```python
from build123d import *

# Parameters (mm, degrees)
SKETCH1_W           = 355.325
SKETCH1_H           = 30
SKETCH1_R           = 12.5
SKETCH1_R_2         = 1
SKETCH1_W_2         = 50
SKETCH1_H_2         = 5
BOSS_EXTRUDE3_DEPTH = 13
FILLET3_R           = 5
SKETCH3_R           = 12.5
BOSS_EXTRUDE4_DEPTH = 13
CUT_EXTRUDE1_REACH  = 359.536
SKETCH4_R           = 1.425
SKETCH5_W           = 63.83
SKETCH5_H           = 18
CUT_EXTRUDE3_DEPTH  = 358.535810269
FILLET4_R           = 5
SKETCH6_W           = 63.8325
SKETCH6_H           = 17
CUT_EXTRUDE4_DEPTH  = 5
SKETCH7_R           = 2.159563788
SKETCH7_R_2         = 1
SKETCH7_R_3         = 2.117135705
SKETCH7_R_4         = 1.916104153
SKETCH7_R_5         = 2.415941568
BOSS_EXTRUDE5_DEPTH = 8
SKETCH8_R           = 12.5
BOSS_EXTRUDE6_DEPTH = 13
SKETCH10_W          = 20
SKETCH10_H          = 10
SKETCH10_R          = 12.5
CUT_EXTRUDE6_DEPTH  = 358.535810269
SKETCH11_R          = 13.25
CUT_EXTRUDE7_DEPTH  = 289.073524686
SKETCH12_R          = 1.25
CUT_EXTRUDE8_DEPTH  = 289.567766088
SKETCH15_R          = 1.6
CUT_EXTRUDE10_DEPTH = 292.788203368
SKETCH17_R          = 4
CUT_EXTRUDE11_DEPTH = 7.5
SKETCH18_R          = 4.25
CUT_EXTRUDE12_DEPTH = 7.5
SKETCH19_W          = 52.537451678
SKETCH19_H          = 17.901984435
CUT_EXTRUDE13_DEPTH = 5
CUT_EXTRUDE14_START = -5
SKETCH20_R          = 12.5
CUT_EXTRUDE14_DEPTH = 5


with BuildPart() as part:
    # Sketch1 → Boss-Extrude3 (new body)
    # profile 1 of 3: a face of its own
    with BuildSketch(Plane.XY):
        with Locations((177.6625, 15)):
            Rectangle(SKETCH1_W, SKETCH1_H)
        with Locations(Location((334.55, 14.5, 0), (0, 0, 180))):
            Circle(SKETCH1_R, mode=Mode.SUBTRACT)
        with Locations(Location((20.775, 14.5, 0), (0, 0, 180))):
            Circle(SKETCH1_R, mode=Mode.SUBTRACT)
    # profile 2 of 3: a face of its own
    with BuildSketch(Plane.XY):
        Polygon((177.6625, 0), (50, 0), (50, -5), (50, -17), (177.6625, -17), align=None)
        with Locations(Location((60, -14.5, 0), (0, 0, 180))):
            Circle(SKETCH1_R_2, mode=Mode.SUBTRACT)
        with Locations(Location((68, -14.5, 0), (0, 0, 180))):
            Circle(SKETCH1_R_2, mode=Mode.SUBTRACT)
        with Locations(Location((60, -2.5, 0), (0, 0, 180))):
            Circle(SKETCH1_R_2, mode=Mode.SUBTRACT)
        with Locations(Location((68, -2.5, 0), (0, 0, 180))):
            Circle(SKETCH1_R_2, mode=Mode.SUBTRACT)
    # profile 3 of 3: a face of its own
    with BuildSketch(Plane.XY):
        with Locations((25, -2.5)):
            Rectangle(SKETCH1_W_2, SKETCH1_H_2)
    extrude(amount=BOSS_EXTRUDE3_DEPTH)

    # Fillet3
    fillet3_edges = [part.edges().sort_by_distance(p)[0] for p in [
        (0, -5, 6.5),
        (0, 30, 6.5),
        (355.325, 30, 6.5),
        (355.325, 0, 6.5),
        (177.6625, -17, 6.5),
        (50, -17, 6.5),
    ]]
    fillet(fillet3_edges, radius=FILLET3_R)

    # Sketch3 → Boss-Extrude4 (add)
    with BuildSketch(Plane.XY.offset(13)):
        with Locations(Location((85, 14.5, 0), (0, 0, 180))):
            Circle(SKETCH3_R)
        with Locations(Location((165, 14.5, 0), (0, 0, 180))):
            Circle(SKETCH3_R)
        with Locations(Location((245, 14.5, 0), (0, 0, 180))):
            Circle(SKETCH3_R)
    extrude(amount=BOSS_EXTRUDE4_DEPTH)

    # Sketch4 → Cut-Extrude1 (cut, up to next)
    with BuildSketch(Plane(origin=(0, 0, 0), x_dir=(-1, 0, 0), z_dir=(0, 0, -1)), mode=Mode.PRIVATE) as cut_extrude1_sk1:
        with Locations((-68, -2.5)):
            Circle(SKETCH4_R)
    cut_extrude1_tool1 = extrude(cut_extrude1_sk1.sketch, amount=-CUT_EXTRUDE1_REACH, mode=Mode.PRIVATE) & part.part
    # Sketch4 → Cut-Extrude1 (cut, up to next)
    with BuildSketch(Plane(origin=(0, 0, 0), x_dir=(-1, 0, 0), z_dir=(0, 0, -1)), mode=Mode.PRIVATE) as cut_extrude1_sk2:
        with Locations((-60, -2.5)):
            Circle(SKETCH4_R)
    cut_extrude1_tool2 = extrude(cut_extrude1_sk2.sketch, amount=-CUT_EXTRUDE1_REACH, mode=Mode.PRIVATE) & part.part
    # Sketch4 → Cut-Extrude1 (cut, up to next)
    with BuildSketch(Plane(origin=(0, 0, 0), x_dir=(-1, 0, 0), z_dir=(0, 0, -1)), mode=Mode.PRIVATE) as cut_extrude1_sk3:
        with Locations((-60, -14.5)):
            Circle(SKETCH4_R)
    cut_extrude1_tool3 = extrude(cut_extrude1_sk3.sketch, amount=-CUT_EXTRUDE1_REACH, mode=Mode.PRIVATE) & part.part
    # Sketch4 → Cut-Extrude1 (cut, up to next)
    with BuildSketch(Plane(origin=(0, 0, 0), x_dir=(-1, 0, 0), z_dir=(0, 0, -1)), mode=Mode.PRIVATE) as cut_extrude1_sk4:
        with Locations((-68, -14.5)):
            Circle(SKETCH4_R)
    cut_extrude1_tool4 = extrude(cut_extrude1_sk4.sketch, amount=-CUT_EXTRUDE1_REACH, mode=Mode.PRIVATE) & part.part
    add(cut_extrude1_tool1.solids().sort_by_distance((68, -2.5, 0))[0], mode=Mode.SUBTRACT)
    add(cut_extrude1_tool2.solids().sort_by_distance((60, -2.5, 0))[0], mode=Mode.SUBTRACT)
    add(cut_extrude1_tool3.solids().sort_by_distance((60, -14.5, 0))[0], mode=Mode.SUBTRACT)
    add(cut_extrude1_tool4.solids().sort_by_distance((68, -14.5, 0))[0], mode=Mode.SUBTRACT)

    # Sketch5 → Cut-Extrude3 (cut, through all)
    with BuildSketch(Plane(origin=(0, 0, 0), x_dir=(-1, 0, 0), z_dir=(0, 0, -1))):
        with Locations((-145.7475, -9)):
            Rectangle(SKETCH5_W, SKETCH5_H)
    extrude(amount=-CUT_EXTRUDE3_DEPTH, mode=Mode.SUBTRACT)

    # Fillet4
    fillet4_edges = [part.edges().sort_by_distance(p)[0] for p in [
        (113.8325, -17, 6.5),
    ]]
    fillet(fillet4_edges, radius=FILLET4_R)

    # Sketch6 → Cut-Extrude4 (cut)
    with BuildSketch(Plane.XY.offset(13)):
        with Locations((81.91625, -8.5)):
            Rectangle(SKETCH6_W, SKETCH6_H)
    extrude(amount=-CUT_EXTRUDE4_DEPTH, mode=Mode.SUBTRACT)

    # Sketch7 → Boss-Extrude5 (add)
    # profile 1 of 4: a face of its own
    with BuildSketch(Plane.XY.offset(8)):
        with Locations((60, -14.5)):
            Circle(SKETCH7_R)
        with Locations((60, -14.5)):
            Circle(SKETCH7_R_2, mode=Mode.SUBTRACT)
    # profile 2 of 4: a face of its own
    with BuildSketch(Plane.XY.offset(8)):
        with Locations((60, -2.5)):
            Circle(SKETCH7_R_3)
        with Locations((60, -2.5)):
            Circle(SKETCH7_R_2, mode=Mode.SUBTRACT)
    # profile 3 of 4: a face of its own
    with BuildSketch(Plane.XY.offset(8)):
        with Locations((68, -2.5)):
            Circle(SKETCH7_R_4)
        with Locations((68, -2.5)):
            Circle(SKETCH7_R_2, mode=Mode.SUBTRACT)
    # profile 4 of 4: a face of its own
    with BuildSketch(Plane.XY.offset(8)):
        with Locations((68, -14.5)):
            Circle(SKETCH7_R_5)
        with Locations((68, -14.5)):
            Circle(SKETCH7_R_2, mode=Mode.SUBTRACT)
    extrude(amount=-BOSS_EXTRUDE5_DEPTH)

    # Sketch8 → Boss-Extrude6 (add)
    with BuildSketch(Plane.XY.offset(26)):
        with Locations(Location((85, 14.5, 0), (0, 0, 180))):
            Circle(SKETCH8_R)
        with Locations(Location((165, 14.5, 0), (0, 0, 180))):
            Circle(SKETCH8_R)
        with Locations(Location((245, 14.5, 0), (0, 0, 180))):
            Circle(SKETCH8_R)
    extrude(amount=BOSS_EXTRUDE6_DEPTH)

    # Sketch10 → Cut-Extrude6 (cut, through all)
    # profile 1 of 2: a face of its own
    with BuildSketch(Plane.XY.offset(13)):
        with Locations((275.325, 15)):
            Rectangle(SKETCH10_W, SKETCH10_H)
    # profile 2 of 2: a face of its own
    with BuildSketch(Plane.XY.offset(13)):
        with BuildLine():
            ThreePointArc((355.325, 25), (353.860533906, 28.535533906), (350.325, 30))
            Line((350.325, 30), (285.325, 30))
            Line((285.325, 30), (285.325, 20))
            Line((285.325, 20), (285.325, 10))
            Line((285.325, 10), (285.325, 0))
            Line((285.325, 0), (350.325, 0))
            ThreePointArc((350.325, 0), (353.860533906, 1.464466094), (355.325, 5))
            Line((355.325, 5), (355.325, 25))
        make_face()
        with Locations((334.55, 14.5)):
            Circle(SKETCH10_R, mode=Mode.SUBTRACT)
    extrude(amount=-CUT_EXTRUDE6_DEPTH, mode=Mode.SUBTRACT)

    # Sketch11 → Cut-Extrude7 (cut, through all)
    with BuildSketch(Plane.XY.offset(13)):
        with Locations((20.775, 14.5)):
            Circle(SKETCH11_R)
    extrude(amount=-CUT_EXTRUDE7_DEPTH, mode=Mode.SUBTRACT)

    # Sketch12 → Cut-Extrude8 (cut, through all)
    with BuildSketch(Plane.XY.offset(8)):
        with Locations((60, -2.5)):
            Circle(SKETCH12_R)
        with Locations((68, -2.5)):
            Circle(SKETCH12_R)
        with Locations((68, -14.5)):
            Circle(SKETCH12_R)
        with Locations((60, -14.5)):
            Circle(SKETCH12_R)
    extrude(amount=-CUT_EXTRUDE8_DEPTH, mode=Mode.SUBTRACT)

    # Sketch15 → Cut-Extrude10 (cut, through all)
    with BuildSketch(Plane(origin=(0, 30, 0), x_dir=(1, 0, 0), z_dir=(0, 1, 0))):
        with Locations(Location((275.325, -6.5, 0), (0, 0, 180))):
            Circle(SKETCH15_R)
    extrude(amount=-CUT_EXTRUDE10_DEPTH, mode=Mode.SUBTRACT)

    # Sketch17 → Cut-Extrude11 (cut)
    with BuildSketch(Plane(origin=(0, 30, 0), x_dir=(1, 0, 0), z_dir=(0, 1, 0))):
        with Locations(Location((275.325, -6.5, 0), (0, 0, 180))):
            Circle(SKETCH17_R)
    extrude(amount=-CUT_EXTRUDE11_DEPTH, mode=Mode.SUBTRACT)

    # Sketch18 → Cut-Extrude12 (cut)
    with BuildSketch(Plane.XZ):
        with Locations(Location((275.325, 6.5, 0), (0, 0, 270))):
            Circle(SKETCH18_R)
    extrude(amount=-CUT_EXTRUDE12_DEPTH, mode=Mode.SUBTRACT)

    # Sketch19 → Cut-Extrude13 (cut)
    with BuildSketch(Plane.XY.offset(13)):
        with Locations((23.731274161, -8.950992218)):
            Rectangle(SKETCH19_W, SKETCH19_H)
    extrude(amount=-CUT_EXTRUDE13_DEPTH, mode=Mode.SUBTRACT)

    # Sketch20 → Cut-Extrude14 (cut)
    with BuildSketch(Plane.XY.offset(39).offset(CUT_EXTRUDE14_START)):
        with Locations(Location((85, 14.5, 0), (0, 0, 180))):
            Circle(SKETCH20_R)
        with Locations(Location((165, 14.5, 0), (0, 0, 180))):
            Circle(SKETCH20_R)
        with Locations(Location((245, 14.5, 0), (0, 0, 180))):
            Circle(SKETCH20_R)
    extrude(amount=CUT_EXTRUDE14_DEPTH, mode=Mode.SUBTRACT)


solid = part.part
```
Check sheet for the modelled part. Datum: model origin and axes. Units: mm. A direction names the side the tool comes from. Coordinates: 2 decimals unless noted, no trailing zeros. Order: outer loops, then holes, each group sorted by start corner. A loop starts at its lowest first (then second) coordinate and runs counter-clockwise, first axis right, second up. Notation, with made-up numbers: (-16, 87.25) -> (0, 87.25) arc R36 ccw to (0, 126.25) -> close; hole circle Ø4 at (-22.5, 67). An arc over 180 degrees is marked (long way). Write each question's results on one line, items separated by ' | '. Start each with the question number.
1) Depth check by flat-ended pin: pin 1 (6.5 mm diameter, centred on x = 275, z = 9, fed in from +Y); pin 2 (7.5 mm diameter, centred on x = 275.325, z = 6.5, fed in from +Y); pin 3 (9 mm diameter, centred on x = 275.325, z = 6.5, fed in from -Y); pin 4 (1 mm diameter, centred on y = 13, z = 3.5, fed in from +X) (3 decimals). Enter the tip coordinate at first touch or a pass-through.
2) Draft check along X on faces 6 (the face through (113.833, -6, 4)), 7 (the face through (50, -8, 4)), 8 (the face through (141, 12, 0)), 9 (the face through (73.453, 19.288, 23.353)). Enter one of: pulls with the +X half, pulls with the -X half, needs draft (parallel to the pull), parting line crosses it, or undercut.
3) Section check D-D (y = -7.5). Enter the section's corners in (x, z), and give its area (3 significant figures).
4) Set-up check for faces 1 (the face through (233, 11, 23)), 2 (the face through (27, -5, 4)), 3 (the face through (172, 0, 8)), 4 (the face through (273, 7.5, 7)), 5 (the face through (265.325, 15, 7)): record each of +Z, -Z, +X, -X, +Y, -Y from which the full face is reachable in a straight line by a thin tool's end or side.
5) Section check B-B (x = 85). Enter the section's corners in (y, z).
6) Section check A-A (y = 14.5). Enter the section's corners in (x, z) (3 decimals).
7) Section check C-C (z = 22.5). Enter the section's corners in (x, y).
8) Material ranges on line 1 along Y through (x, z) = (68, 4); line 2 along X through (y, z) = (4.5, 6.5) (3 decimals); line 3 along X through (y, z) = (4.25, 6.5) (3 decimals), recorded low to high.
Checked values:
1) pin 1: y = 30 | pin 2: y = 22.5 | pin 3: y = 0 | pin 4: x = 265.325
2) face 6: pulls with the +X half | face 7: pulls with the -X half | face 8: needs draft | face 9: undercut
3) outline: (50, 0) -> (113.83, 0) -> (113.83, 8) -> (50, 8) -> close | area: 511 mm²
4) face 1: +Z | face 2: +Z, -Z, -X, -Y | face 3: +Z, +X, -Y | face 4: -Y | face 5: +Z, -Z, +X
5) outline: (-17, 0) -> (30, 0) -> (30, 13) -> (27, 13) -> (27, 34) -> (2, 34) -> (2, 13) -> (0, 13) -> (0, 8) -> (-17, 8) -> close
6) outline: (0, 0) -> (7.525, 0) -> (7.525, 13) -> (0, 13) -> close; (34.025, 0) -> (265.325, 0) -> (265.325, 13) -> (257.5, 13) -> (257.5, 34) -> (232.5, 34) -> (232.5, 13) -> (177.5, 13) -> (177.5, 34) -> (152.5, 34) -> (152.5, 13) -> (97.5, 13) -> (97.5, 34) -> (72.5, 34) -> (72.5, 13) -> (34.025, 13) -> close
7) outline: circle Ø25 at (85, 14.5); circle Ø25 at (165, 14.5); circle Ø25 at (245, 14.5)
8) line 1: -17 to -15.75, -13.25 to -3.75, -1.25 to 30 | line 2: 0 to 12.082, 29.468 to 271.075, 279.575 to 285.325 | line 3: 0 to 12.379, 29.171 to 271.075, 279.575 to 285.325
